from build123d import *

# Parameters (mm, degrees)
EXTRUDE_1_DEPTH     = 6
SKETCH_2_R          = 1.35
CUT_EXTRUDE_1_DEPTH = 6
FILLET_1_R          = 10
SKETCH_3_R          = 1.6
CUT_EXTRUDE_2_DEPTH = 6


with BuildPart() as part:
    # 草图1 → 凸台-拉伸1 (new body)
    with BuildSketch(Plane(origin=(0, 0, 0), x_dir=(1, 0, 0), z_dir=(0, 1, 0))):
        with BuildLine():
            Line((-9.716498114, 14.55471279), (-45, -9))
            Line((-45, -9), (-45, -24))
            Line((-45, -24), (45, -24))
            Line((45, -24), (45, -9))
            Line((45, -9), (9.716498114, 14.55471279))
            ThreePointArc((9.716498114, 14.55471279), (0, 17.5), (-9.716498114, 14.55471279))
        make_face()
    extrude(amount=EXTRUDE_1_DEPTH)

    # 草图2 → 切除-拉伸1 (cut)
    with BuildSketch(Plane(origin=(0, 6, 0), x_dir=(1, 0, 0), z_dir=(0, 1, 0))):
        with Locations(Location((0, 13.5, 0), (0, 0, 270))):
            Circle(SKETCH_2_R)
        with Locations(Location((11.691342951, 6.75, 0), (0, 0, 270))):
            Circle(SKETCH_2_R)
        with Locations(Location((11.691342951, -6.75, 0), (0, 0, 270))):
            Circle(SKETCH_2_R)
        with Locations(Location((0, -13.5, 0), (0, 0, 270))):
            Circle(SKETCH_2_R)
        with Locations(Location((-11.691342951, -6.75, 0), (0, 0, 270))):
            Circle(SKETCH_2_R)
        with Locations(Location((-11.691342951, 6.75, 0), (0, 0, 270))):
            Circle(SKETCH_2_R)
    extrude(amount=-CUT_EXTRUDE_1_DEPTH, mode=Mode.SUBTRACT)

    # 圆角1
    fillet_1_edges = [part.edges().sort_by_distance(p)[0] for p in [
        (45, 3, 9),
        (-45, 3, 9),
    ]]
    fillet(fillet_1_edges, radius=FILLET_1_R)

    # 草图3 → 切除-拉伸2 (cut)
    with BuildSketch(Plane.XZ):
        with Locations(Location((-35, 13, 0), (0, 0, 270))):
            Circle(SKETCH_3_R)
        with Locations(Location((35, 13, 0), (0, 0, 90))):
            Circle(SKETCH_3_R)
    extrude(amount=-CUT_EXTRUDE_2_DEPTH, mode=Mode.SUBTRACT)


solid = part.part
Verification items for the finished model (mm, model axes). Round coordinates to 2 decimals unless told otherwise and drop trailing zeros. Loops run counter-clockwise (first coordinate to the right, second up) from the corner with the lowest first, then second, coordinate; pieces in that order, holes last. Notation, with made-up numbers: (73, -9.5) - (128, -9.5) arc R19 ccw to (128, 24.5) - close; hole circle Ø11 at (41, 62). An arc over 180 degrees is marked (long way). Use a Markdown table: item, result. Add a question column.
1. Thickness scan on probe 1 along X at (y, z) = (3, -6.75); probe 2 along X at (y, z) = (1.7, 13.5); probe 3 along X at (y, z) = (3.7, 13). Record the ranges inside material, lowest first. Write a range as [from, to].
2. Section check C-C, the plane y = 3.35. Give the number of separate pieces and of enclosed holes in the cut face, plus the area to 3 significant figures.
3. Section check D-D, the plane x = -35. Record the boundary of the cut face in (y, z).
4. Release check for a two-part mould opening along X. For faces 1 (the face through (43.8, 3, 9.6)), 2 (the face through (-1, 0, 8)), 3 (the face through (0.06, 3.04, -14.85)) record: released by +X, released by -X, zero draft, split by the parting line, or undercut.
5. Section check B-B, the plane z = -6.75. Record the boundary of the cut face in (x, y).
6. Section check A-A, the plane x = 0. Record the boundary of the cut face in (y, z), plus the area to 3 significant figures.
7. Gauge pin test, flat ends, axial feed: pin 1 (3 mm diameter, centred on x = -7.5, z = 14.5, fed in from -Y); pin 2 (3 mm diameter, centred on y = 2.5, z = 3.5, fed in from +X); pin 3 (1 mm diameter, centred on y = 2, z = 7.5, fed in from -X); pin 4 (1.5 mm diameter, centred on x = -21.5, y = 1.5, fed in from -Z). Record the tip position at first contact, or that the pin passes through.
Checks:
| question | item | result |
|---|---|---|
| 1 | probe 1 | x = [-21.41, -13.04], [-10.34, 10.34], [13.04, 21.41] |
| 1 | probe 2 | x = [-44.96, -36.52], [-33.48, -1.35], [1.35, 33.48], [36.52, 44.96] |
| 1 | probe 3 | x = [-44.91, -36.6], [-33.4, -1.25], [1.25, 33.4], [36.6, 44.91] |
| 2 | separate pieces | 1 |
| 2 | enclosed holes | 8 |
| 2 | area | 2,620 mm^2 |
| 3 | outline | (0, 2.32) - (6, 2.32) - (6, 11.4) - (0, 11.4) - close; (0, 14.6) - (6, 14.6) - (6, 24) - (0, 24) - close |
| 4 | face 1 | released by +X |
| 4 | face 2 | zero draft |
| 4 | face 3 | undercut |
| 5 | outline | (-21.41, 0) - (-13.04, 0) - (-13.04, 6) - (-21.41, 6) - close; (-10.34, 0) - (10.34, 0) - (10.34, 6) - (-10.34, 6) - close; (13.04, 0) - (21.41, 0) - (21.41, 6) - (13.04, 6) - close |
| 6 | outline | (0, -17.5) - (6, -17.5) - (6, -14.85) - (0, -14.85) - close; (0, -12.15) - (6, -12.15) - (6, 12.15) - (0, 12.15) - close; (0, 14.85) - (6, 14.85) - (6, 24) - (0, 24) - close |
| 6 | area | 217 mm^2 |
| 7 | pin 1 | stops at y = 0 |
| 7 | pin 2 | stops at x = 39.01 |
| 7 | pin 3 | stops at x = -42.73 |
| 7 | pin 4 | stops at z = -7.19 |
